from build123d import *

# Parameters (mm, degrees)
CORTAR_EXTRUIR1_START = -1.8
CORTAR_EXTRUIR1_DEPTH = 3


with BuildPart() as part:
    # Croquis1 → Revolución1 (revolve)
    with BuildSketch(Plane.XY):
        with BuildLine():
            Line((0, 0), (0, 11.9))
            ThreePointArc((0, 11.9), (1.726548348, 11.569000929), (3.231811568, 10.660864252))
            ThreePointArc((3.231811568, 10.660864252), (3.282156956, 10.593022088), (3.3, 10.5104458))
            Line((3.3, 10.5104458), (3.3, 9.7))
            ThreePointArc((3.3, 9.7), (3.241421356, 9.558578644), (3.1, 9.5))
            Line((3.1, 9.5), (1.6, 9.5))
            Line((1.6, 9.5), (1.6, 2.771281292))
            Line((1.6, 2.771281292), (0, 0))
        make_face()
    revolve(axis=Axis((0, 0, 0), (0, 1, 0)))

    # Croquis2 → Cortar-Extruir1 (cut)
    with BuildSketch(Plane.XZ.offset(-9.5).offset(CORTAR_EXTRUIR1_START)):
        with BuildLine():
            Line((-0.4, 3.2), (-0.4, 0.9))
            ThreePointArc((-0.4, 0.9), (-0.546446609, 0.546446609), (-0.9, 0.4))
            Line((-0.9, 0.4), (-3.2, 0.4))
            Line((-3.2, 0.4), (-3.2, -0.4))
            Line((-3.2, -0.4), (-0.9, -0.4))
            ThreePointArc((-0.9, -0.4), (-0.546446609, -0.546446609), (-0.4, -0.9))
            Line((-0.4, -0.9), (-0.4, -3.2))
            Line((-0.4, -3.2), (0.4, -3.2))
            Line((0.4, -3.2), (0.4, -0.9))
            ThreePointArc((0.4, -0.9), (0.546446609, -0.546446609), (0.9, -0.4))
            Line((0.9, -0.4), (3.2, -0.4))
            Line((3.2, -0.4), (3.2, 0.4))
            Line((3.2, 0.4), (0.9, 0.4))
            ThreePointArc((0.9, 0.4), (0.546446609, 0.546446609), (0.4, 0.9))
            Line((0.4, 0.9), (0.4, 3.2))
            Line((0.4, 3.2), (-0.4, 3.2))
        make_face()
    extrude(amount=-CORTAR_EXTRUIR1_DEPTH, mode=Mode.SUBTRACT)


solid = part.part
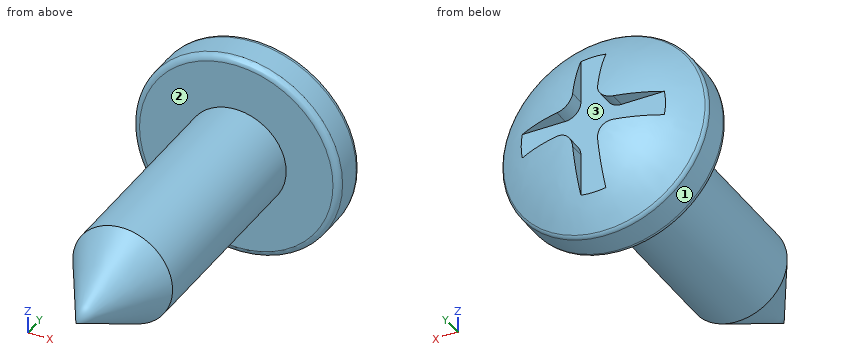
Design review of the part built by this model. Coordinates are the model's own, in mm. Face numbers are marked on the shaded views. Coordinates: 2 decimals unless noted, no trailing zeros. Order: outer loops, then holes, each group sorted by start corner. A loop starts at its lowest first (then second) coordinate and runs counter-clockwise, first axis right, second up.
Item 1: The part is to be moulded in two halves that separate along X. For the marked faces 1, 2 and 3, say which applies: pulls with the +X half, pulls with the -X half, needs draft (parallel to the pull), parting line crosses it, or undercut.
Item 2: Take a section at B-B, the plane y = 2.25. Write out the cut boundary in (x, z), then the cut area to 3 significant figures.
Item 3: For line 1 (X direction, y = 5.5, z = 0); line 2 (Y direction, x = -2.25, z = -0.25); line 3 (Z direction, x = -0.5, y = 2.25), list the stretches that pass through material, from the lowest coordinate up.
Item 4: For pin 1 Ø1.4 at (x, z) = (-1, 0) entering from +Y; pin 2 Ø1 at (x, y) = (0, 5) entering from +Z; pin 3 Ø3 at (x, y) = (0.5, 7.5) entering from -Z; pin 4 Ø0.5 at (x, y) = (1.5, 11.5) entering from +Z, all flat-tipped, find the tip position at first contact; note any pin that passes through.
Item 5: Take a section at A-A, the plane y = 8.5. Write out the cut boundary in (x, z).
The answers:
1. face 1: parting line crosses it
1. face 2: needs draft
1. face 3: undercut
2. outline: circle Ø2.6 at (0, 0)
2. area: 5.30 mm2
3. line 1: x = -1.6 to 1.6
3. line 2: y = 9.5 to 11.3
3. line 3: z = -1.2 to 1.2
4. pin 1: stops at y = 11.83
4. pin 2: stops at z = 1.6
4. pin 3: stops at z = -1.6
4. pin 4: stops at z = 1.91
5. outline: circle Ø3.2 at (0, 0)
